Source: three-view drawing plus pictorial views. Frame: mm from the lowest corner of the part. A direction names the side the tool comes from. Give positions to 0.01 mm unless a question says otherwise; leave off trailing zeros. Write each loop counter-clockwise with the first axis right and the second up, starting at its lowest first coordinate (ties: lowest second). Pieces come first, ordered by that corner, then holes.
Q1. Reachability of the marked faces 1 and 2 from +Z, -Z, +X, -X, +Y, -Y: full face, straight path, thin tool, end or side. Return the list, or none.
Q2. Cut plane D-D on x = 3.5. Return the cut outline in (y, z).
Q3. Pin query (flat end, axial travel): pin 1 (5 mm diameter, centred on x = 14, y = 9, fed in from -Z); pin 2 (3 mm diameter, centred on x = 17, z = 2.5, fed in from +Y). Return the tip coordinate at first contact, or that it passes through.
Q4. Cut plane A-A on z = 5. Return the cut outline in (x, y), plus the area to 3 significant figures.
Q5. Cut plane C-C on y = 6. Return the cut outline in (x, z), plus the area to 3 significant figures.
Q6. Line query: L1, parallel to X at y = 0.2, z = 5; L2, parallel to Y at x = 8, z = 12.3; L3, parallel to Y at x = 3.5, z = 12.4. Output: solid intervals per line, ascending.
Q7. Cut plane B-B on x = 17. Return the cut outline in (y, z), plus the area to 3 significant figures.
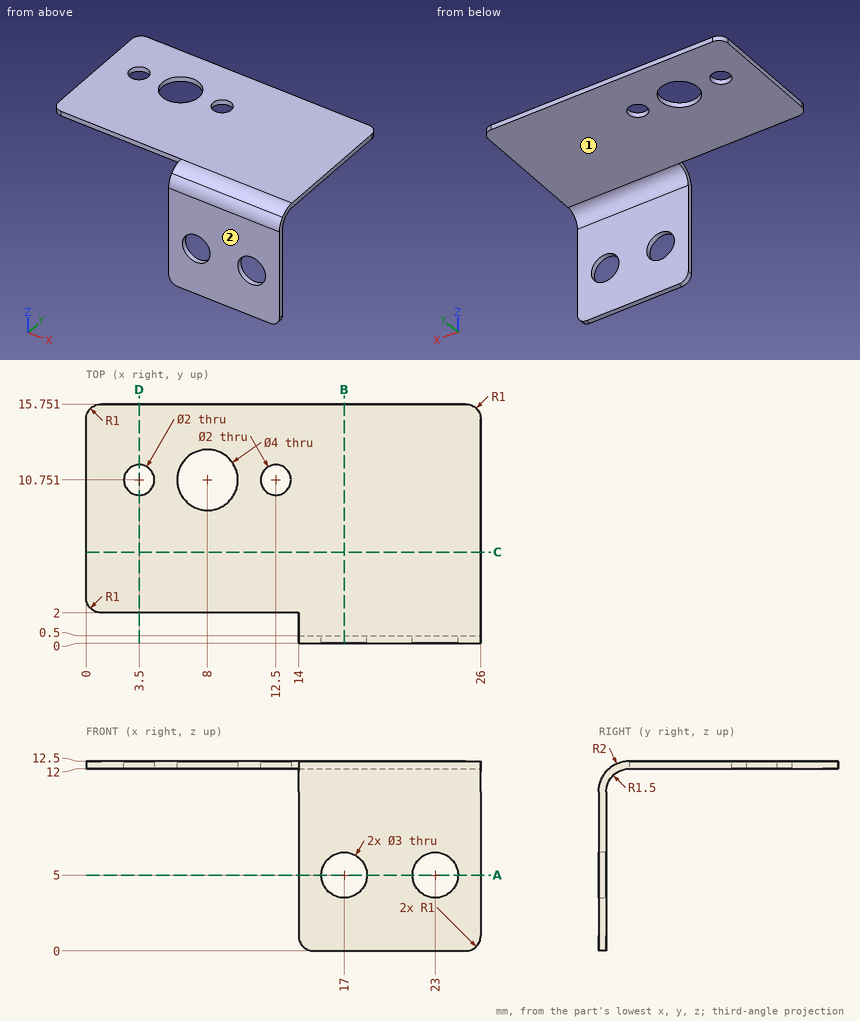
Data:
1. face 1: -Z, +X, -X, +Y
1. face 2: +Z, -Z, +X, -X, -Y
2. outline: (2, 12) - (9.75, 12) - (9.75, 12.5) - (2, 12.5) - close; (11.75, 12) - (15.75, 12) - (15.75, 12.5) - (11.75, 12.5) - close
3. pin 1: stops at z = 12
3. pin 2: stops at y = 0.5
4. outline: (14, 0) - (15.5, 0) - (15.5, 0.5) - (14, 0.5) - close; (18.5, 0) - (21.5, 0) - (21.5, 0.5) - (18.5, 0.5) - close; (24.5, 0) - (26, 0) - (26, 0.5) - (24.5, 0.5) - close
4. area: 3.00 mm2
5. outline: (0, 12) - (26, 12) - (26, 12.5) - (0, 12.5) - close
5. area: 13.0 mm2
6. L1: x = 14 to 15.5, 18.5 to 21.5, 24.5 to 26
6. L2: y = 2 to 8.75, 12.75 to 15.75
6. L3: y = 2 to 9.75, 11.75 to 15.75
7. outline: (0, 0) - (0.5, 0) - (0.5, 3.5) - (0, 3.5) - close; (0, 6.5) - (0.5, 6.5) - (0.5, 10.5) arc R1.5 cw to (2, 12) - (15.75, 12) - (15.75, 12.5) - (2, 12.5) arc R2 ccw to (0, 10.5) - close
7. area: 12.0 mm2
